The model under review builds one solid part; all positions refer to its coordinate system, in mm. A direction names the side the tool comes from. Round coordinates to 2 decimals unless told otherwise and drop trailing zeros. Order: outer loops, then holes, each group sorted by start corner. A loop starts at its lowest first (then second) coordinate and runs counter-clockwise, first axis right, second up. Notation, with made-up numbers: M 65.25,9.5 L 93.25,9.5 A30 ccw 93.25,35.5 Z; hole C 44,55 d9. An arc over 180 degrees is marked long. Answer as a JSON object with one key per item and string values. Group by question number.
1) Consider section B-B, the plane z = -31. Write out the cut boundary in (x, y), then the cut area to 3 significant figures.
2) Insertion check: pin 1 Ø10.5 at (x, y) = (38.1, 16.764) entering from -Z; pin 2 Ø2 at (x, y) = (36.5, 29.5) entering from -Z; pin 3 Ø6 at (x, y) = (21, 20) entering from -Z. Each pin has a flat end and moves straight along its axis. Give the tip position at first contact, or say it passes through.
3) The part is to be moulded in two halves that separate along X. For faces 1 (the flat face through (8.33, 30.28, -20.89)), 2 (the cylindrical face through (14.776, 12.772, -2.218)), 3 (the flat face through (35, 13, -4.5)), 4 (the flat face through (42.7, 3.16, -20.57)), say which applies: +X half, -X half, draft (parallel to the pull), parting line (faces both ways), or undercut.
4) Consider section D-D, the plane y = 14. Write out the cut boundary in (x, z), then the cut area to 3 significant figures.
5) Consider section C-C, the plane x = 40.5. Write out the cut boundary in (y, z), then the cut area to 3 significant figures.
6) To check wall thickness, follow line 1 (Y direction, x = 12.7, z = -6.3); line 2 (Y direction, x = 6, z = -13); line 3 (X direction, y = 23, z = -8.5). State the ranges of each line that lie inside material, in increasing order.
7) For faces 5 (the flat face through (26, 17, -9.5)), 6 (the flat face through (0, 17, -5)), 7 (the flat face through (9, 13, -4.5)), list the 3-axis set-ups (+Z, -Z, +X, -X, +Y, -Y) from which the entire face can be reached by the end or side of a thin tool; tool diameter is ignored.
8) Consider section A-A, the plane x = 25.4. Write out the cut boundary in (y, z), then the cut area to 3 significant figures.
```python
from build123d import *

# Parameters (mm, degrees)
SKETCH1_R                               = 4.7625
BOSS_EXTRUDE1_DEPTH                     = 33.528
CUT_EXTRUDE1_DEPTH                      = 71.978373046
CBORE_FOR_M8_HEX_HEAD_BOLT1_D           = 9
CBORE_FOR_M8_HEX_HEAD_BOLT1_CBORE_D     = 16
CBORE_FOR_M8_HEX_HEAD_BOLT1_CBORE_DEPTH = 5


with BuildPart() as part:
    # Sketch1 → Boss-Extrude1 (new body)
    with BuildSketch(Plane(origin=(0, 0, 0), x_dir=(1, 0, 0), z_dir=(0, 1, 0))):
        with BuildLine():
            Line((0, 0), (50.8, 0))
            Line((50.8, 0), (50.8, 9.4996))
            Line((50.8, 9.4996), (34.368896597, 31.960986975))
            ThreePointArc((34.368896597, 31.960986975), (25.4, 36.5125), (16.431103403, 31.960986975))
            Line((16.431103403, 31.960986975), (0, 9.4996))
            Line((0, 9.4996), (0, 0))
        make_face()
        with Locations(Location((25.4, 25.4, 0), (0, 0, 270))):
            Circle(SKETCH1_R, mode=Mode.SUBTRACT)
    extrude(amount=BOSS_EXTRUDE1_DEPTH)

    # Sketch2 → Cut-Extrude1 (cut, through all)
    with BuildSketch(Plane(origin=(50.8, 0, 0), x_dir=(0, 0, -1), z_dir=(1, 0, 0))):
        Polygon((9.4996, 16.764), (9.4996, 27.1145), (36.5125, 27.1145), (36.5125, 6.4135), (9.4996, 6.4135), align=None)
    extrude(amount=-CUT_EXTRUDE1_DEPTH, mode=Mode.SUBTRACT)

    # CBORE for M8 Hex Head Bolt1 (through all)
    with Locations(Plane(origin=(0, 0, -9.4996), x_dir=(-1, 0, 0), z_dir=(0, 0, -1))):
        with Locations((-12.7, 16.764), (-38.1, 16.764)):
            CounterBoreHole(CBORE_FOR_M8_HEX_HEAD_BOLT1_D / 2, CBORE_FOR_M8_HEX_HEAD_BOLT1_CBORE_D / 2, CBORE_FOR_M8_HEX_HEAD_BOLT1_CBORE_DEPTH)


solid = part.part
```
Results list:
{
 "1": {"outline": "M 15.73,0 L 35.07,0 L 35.07,6.41 L 15.73,6.41 Z; M 15.73,27.11 L 35.07,27.11 L 35.07,33.53 L 15.73,33.53 Z", "area": "248 mm^2"},
 "2": {"pin 1": "z = -4.5", "pin 2": "z = -30.41", "pin 3": "z = -9.5"},
 "3": {"face 1": "-X half", "face 2": "undercut", "face 3": "undercut", "face 4": "+X half"},
 "4": {"outline": "M 0,-9.5 L 5.19,-9.5 L 5.19,-4.5 L 9.15,-4.5 L 9.15,0 L 0,0 Z; M 16.25,-4.5 L 20.21,-4.5 L 20.21,-9.5 L 30.59,-9.5 L 30.59,-4.5 L 34.55,-4.5 L 34.55,0 L 16.25,0 Z; M 41.65,-4.5 L 45.61,-4.5 L 45.61,-9.5 L 50.8,-9.5 L 50.8,0 L 41.65,0 Z", "area": "269 mm^2"},
 "5": {"outline": "M 0,-23.58 L 6.41,-23.58 L 6.41,-9.5 L 9.13,-9.5 L 9.13,-4.5 L 12.96,-4.5 L 12.96,0 L 0,0 Z; M 20.57,-4.5 L 24.4,-4.5 L 24.4,-9.5 L 27.11,-9.5 L 27.11,-23.58 L 33.53,-23.58 L 33.53,0 L 20.57,0 Z", "area": "389 mm^2"},
 "6": {"line 1": "0 to 8.76, 24.76 to 33.53", "line 2": "0 to 6.41, 27.11 to 33.53", "line 3": "0 to 7.69, 17.71 to 33.09, 43.11 to 50.8"},
 "7": {"face 5": "-Z, +X, -X", "face 6": "+Z, -Z, -X, +Y, -Y", "face 7": "-Z"},
 "8": {"outline": "M 0,-36.51 L 6.41,-36.51 L 6.41,-30.16 L 0,-30.16 Z; M 0,-20.64 L 6.41,-20.64 L 6.41,-9.5 L 27.11,-9.5 L 27.11,-20.64 L 33.53,-20.64 L 33.53,0 L 0,0 Z; M 27.11,-36.51 L 33.53,-36.51 L 33.53,-30.16 L 27.11,-30.16 Z", "area": "543 mm^2"}
}
